The model under review builds one solid part; all positions refer to its coordinate system, in mm. A direction names the side the tool comes from. Give positions to 0.01 mm unless a question says otherwise; leave off trailing zeros. Order: outer loops, then holes, each group sorted by start corner. A loop starts at its lowest first (then second) coordinate and runs counter-clockwise, first axis right, second up.
```python
from build123d import *

# Parameters (mm, degrees)
SKETCH2_W           = 51.2
SKETCH2_H           = 53.4
BOSS_EXTRUDE2_DEPTH = 2.5
SKETCH3_R           = 40.2
BOSS_EXTRUDE3_DEPTH = 2.5
SKETCH4_R           = 2.5
BOSS_EXTRUDE4_DEPTH = 10
SKETCH5_W           = 5.8
SKETCH5_H           = 8
BOSS_EXTRUDE5_DEPTH = 8
SKETCH6_R           = 1.25
SKETCH6_R_2         = 1.7
CUT_EXTRUDE1_DEPTH  = 83.714750801
SKETCH7_R           = 2.1
CUT_EXTRUDE2_DEPTH  = 5.2
SKETCH8_W           = 4
SKETCH8_H           = 12.6
BOSS_EXTRUDE6_DEPTH = 13.3


with BuildPart() as part:
    # Sketch2 → Boss-Extrude2 (new body)
    with BuildSketch(Plane.XY.offset(6)):
        with Locations((-45.6, 0)):
            Rectangle(SKETCH2_W, SKETCH2_H)
    extrude(amount=BOSS_EXTRUDE2_DEPTH)

    # Sketch3 → Boss-Extrude3 (add)
    with BuildSketch(Plane.XY.offset(6)):
        Circle(SKETCH3_R)
    extrude(amount=BOSS_EXTRUDE3_DEPTH)

    # Sketch4 → Boss-Extrude4 (add)
    with BuildSketch(Plane.XY.offset(8.5)):
        with Locations((-54.2, -24.17)):
            Circle(SKETCH4_R)
        with Locations((-53, 24.13)):
            Circle(SKETCH4_R)
        with Locations((-2.2, -19.07)):
            Circle(SKETCH4_R)
        with Locations((-2.2, 8.93)):
            Circle(SKETCH4_R)
    extrude(amount=BOSS_EXTRUDE4_DEPTH)

    # Sketch5 → Boss-Extrude5 (add)
    with BuildSketch(Plane.XY.offset(8.5)):
        with Locations((-68.3, -5)):
            Rectangle(SKETCH5_W, SKETCH5_H)
    extrude(amount=BOSS_EXTRUDE5_DEPTH)

    # Sketch6 → Cut-Extrude1 (cut, through all)
    with BuildSketch(Plane.XY.offset(6)):
        with Locations((-54.2, -24.17)):
            Circle(SKETCH6_R)
        with Locations((-53, 24.13)):
            Circle(SKETCH6_R)
        with Locations((-2.2, -19.07)):
            Circle(SKETCH6_R)
        with Locations((-2.2, 8.93)):
            Circle(SKETCH6_R)
        with Locations((28, 28)):
            Circle(SKETCH6_R_2)
        with Locations((28, -28)):
            Circle(SKETCH6_R_2)
    extrude(amount=CUT_EXTRUDE1_DEPTH, mode=Mode.SUBTRACT)

    # Sketch7 → Cut-Extrude2 (cut)
    with BuildSketch(Plane(origin=(-71.2, 0, 0), x_dir=(0, 0, -1), z_dir=(1, 0, 0))):
        with Locations((-12.5, -5)):
            Circle(SKETCH7_R)
    extrude(amount=CUT_EXTRUDE2_DEPTH, mode=Mode.SUBTRACT)

    # Sketch8 → Boss-Extrude6 (add)
    with BuildSketch(Plane.XY.offset(6)):
        with Locations((-72.5, 11.4)):
            Rectangle(SKETCH8_W, SKETCH8_H)
    extrude(amount=BOSS_EXTRUDE6_DEPTH)


solid = part.part
```
1. For faces 5 (the flat face through (-73, 5.1, 13)), 6 (the flat face through (-70.5, 11, 14)), 7 (the flat face through (-68, -9, 12)), 8 (the flat face through (-66, -5, 13)), list the 3-axis set-ups (+Z, -Z, +X, -X, +Y, -Y) from which the entire face can be reached by the end or side of a thin tool; tool diameter is ignored.
2. Take a section at D-D (x = -62.5). Write out the cut boundary in (y, z), and give its area (4 significant figures).
3. Insertion check: pin 1 (6 mm diameter, centred on y = -13, z = 9, fed in from -X); pin 2 (0.8 mm diameter, centred on x = -44, z = 7, fed in from -Y); pin 3 (1.2 mm diameter, centred on x = -72, z = 11.5, fed in from -Y). Each pin has a flat end and moves straight along its axis. Give the tip position at first contact, or say it passes through.
4. Take a section at A-A (z = 12.5). Count the separate pieces of the cut face and the enclosed holes in it, and give its area (3 significant figures).
5. Take a section at B-B (y = 8.93). Write out the cut boundary in (x, z).
6. To check wall thickness, follow line 1 (Z direction, x = 26.5, y = -19.5); line 2 (Y direction, x = -69, z = 7); line 3 (Y direction, x = 28, z = 6.6). State the ranges of each line that lie inside material, in increasing order.
7. Draft analysis for pull direction Y (two halves, no side actions). For faces 1 (the flat face through (-51, -26.7, 7)), 2 (the cylindrical face through (-3.45, 8.98, 12.16)), 3 (the cylindrical face through (-2.36, -17.83, 12.16)), 4 (the flat face through (-1, 8, 18.5)), state which applies: pulls with the +Y half, pulls with the -Y half, needs draft (parallel to the pull), parting line crosses it, or undercut.
8. Take a section at C-C (x = -2.2). Write out the cut boundary in (y, z), and give its area (3 significant figures).
Answer:
1. face 5: +Z, -X
1. face 6: +Z, +Y
1. face 7: +Z, +X, -X, -Y
1. face 8: -X
2. outline: (-26.7, 6) - (26.7, 6) - (26.7, 8.5) - (-26.7, 8.5) - close
2. area: 133.5 mm2
3. pin 1: stops at x = -71.2
3. pin 2: stops at y = -26.7
3. pin 3: stops at y = 5.1
4. separate pieces: 6
4. enclosed holes: 4
4. area: 134 mm2
5. outline: (-74.5, 6) - (-3.45, 6) - (-3.45, 18.5) - (-4.7, 18.5) - (-4.7, 8.5) - (-70.5, 8.5) - (-70.5, 19.3) - (-74.5, 19.3) - close; (-0.95, 6) - (39.2, 6) - (39.2, 8.5) - (0.3, 8.5) - (0.3, 18.5) - (-0.95, 18.5) - close
6. line 1: z = 6 to 8.5
6. line 2: y = -26.7 to 26.7
6. line 3: y = -26.3 to 26.3
7. face 1: pulls with the -Y half
7. face 2: undercut
7. face 3: undercut
7. face 4: needs draft
8. outline: (-40.14, 6) - (-20.32, 6) - (-20.32, 18.5) - (-21.57, 18.5) - (-21.57, 8.5) - (-40.14, 8.5) - close; (-17.82, 6) - (7.68, 6) - (7.68, 18.5) - (6.43, 18.5) - (6.43, 8.5) - (-16.57, 8.5) - (-16.57, 18.5) - (-17.82, 18.5) - close; (10.18, 6) - (40.14, 6) - (40.14, 8.5) - (11.43, 8.5) - (11.43, 18.5) - (10.18, 18.5) - close
8. area: 238 mm2
